from build123d import *

# Parameters (mm, degrees)
BOSS_EXTRUDE1_DEPTH      = 2
BOSS_EXTRUDE1_DEPTH_BACK = 2
SKETCH2_R                = 4
SKETCH2_R_2              = 2.5
SKETCH4_R                = 2
BOSS_EXTRUDE2_DEPTH      = 4
BOSS_EXTRUDE3_DEPTH      = 2


with BuildPart() as part:
    # Sketch2 → Boss-Extrude1 (new, two sides: drawn at the far end of the back side and taken through both)
    with BuildSketch(Plane(origin=(0, 0, 0), x_dir=(1, 0, 0), z_dir=(0, 1, 0)).offset(-BOSS_EXTRUDE1_DEPTH_BACK)):
        Polygon((-52.5, 10), (52.5, 10), (52.5, 0), (52.5, -2.5), (47.5, -7.5), (42.5, -7.5), (32.5, 2.5), (17.5, 2.5), (7.5, -7.5), (-7.5, -7.5), (-17.5, 2.5), (-32.5, 2.5), (-42.5, -7.5), (-47.5, -7.5), (-52.5, -2.5), (-52.5, 0), align=None)
        with Locations(Location((0, 0, 0), (0, 0, 270))):
            Circle(SKETCH2_R, mode=Mode.SUBTRACT)
        with Locations(Location((-45, 0, 0), (0, 0, 270))):
            Circle(SKETCH2_R_2, mode=Mode.SUBTRACT)
        with Locations(Location((45, 0, 0), (0, 0, 90))):
            Circle(SKETCH2_R_2, mode=Mode.SUBTRACT)
    extrude(amount=BOSS_EXTRUDE1_DEPTH + BOSS_EXTRUDE1_DEPTH_BACK)

    # Sketch4 → Boss-Extrude2 (add)
    with BuildSketch(Plane(origin=(0, 0, -10), x_dir=(-1, 0, 0), z_dir=(0, 0, -1))):
        Polygon((52.5, -8), (42.25, -8), (32.25, -18), (20.25, -18), (10.25, -8), (-10.25, -8), (-20.25, -18), (-32.25, -18), (-42.25, -8), (-52.5, -8), (-52.5, 8), (-42.25, 8), (-32.25, 18), (-20.25, 18), (-10.25, 8), (10.25, 8), (20.25, 18), (32.25, 18), (42.25, 8), (52.5, 8), align=None)
        with Locations((26.25, -10.674724776)):
            Circle(SKETCH4_R, mode=Mode.SUBTRACT)
        with Locations(Location((-26.25, -10.674724776, 0), (0, 0, 180))):
            Circle(SKETCH4_R, mode=Mode.SUBTRACT)
        with Locations((-26.25, 10.674724776)):
            Circle(SKETCH4_R, mode=Mode.SUBTRACT)
        with Locations(Location((26.25, 10.674724776, 0), (0, 0, 180))):
            Circle(SKETCH4_R, mode=Mode.SUBTRACT)
    extrude(amount=BOSS_EXTRUDE2_DEPTH)

    # Sketch5 → Boss-Extrude3 (add)
    with BuildSketch(Plane.ZY.offset(17.5)):
        Polygon((-10, 7), (-10, 2), (-2.5, 2), align=None)
        Polygon((-2.5, -2), (-10, -7), (-10, -2), align=None)
    boss_extrude3 = extrude(amount=-BOSS_EXTRUDE3_DEPTH)

    # Mirror1: Boss-Extrude3 across plane
    add(boss_extrude3.mirror(Plane(origin=(0, 0, 0), x_dir=(0, 0, 1), z_dir=(1, 0, 0))))


solid = part.part
Here's how the part is built. I have some questions about the finished solid (model axes, mm). A direction names the side the tool comes from. Give positions to 0.01 mm unless a question says otherwise; leave off trailing zeros. Write each loop counter-clockwise with the first axis right and the second up, starting at its lowest first coordinate (ties: lowest second). Pieces come first, ordered by that corner, then holes. Notation, with made-up numbers: (83.5, 7.25) -> (109.5, 7.25) arc R13 cw to (109.5, 28.25) -> close; hole circle Ø2 at (14, -15.75). An arc over 180 degrees is marked (long way). Use one line per item in the form item = value. Start each with the question number.
1. Imagine slicing it at A-A on x = -45. List the corners of the cut face in (y, z) for me, plus the area to 3 significant figures.
2. On a 3-axis mill with a long thin cutter (end or side, diameter ignored), from which of +Z, -Z, +X, -X, +Y, -Y can I reach the whole of each face in a straight line? I mean faces 5 (the face through (-39, 2, -3)), 6 (the face through (39, -2, -3)), 7 (the face through (25, 0, -2.5)). Say none if no direction works.
3. Imagine slicing it at D-D on x = -26.25. List the corners of the cut face in (y, z) for me, plus the area to 3 significant figures.
4. If I drill on L1, parallel to Y at x = -26.25, z = -11.3; L2, parallel to Z at x = 45, y = -1; L3, parallel to Z at x = -40, y = 4, over which ranges is the centre line in solid material (lowest first)?
5. Thinking about a two-plate mould opening in Y: for faces 1 (the face through (15.32, 13.07, -11.97)), 2 (the face through (45, 0, 7.5)), 3 (the face through (-16.514, -4.465, -6.198)), 4 (the face through (24.342, 11.275, -11.972)), which applies, +Y half, -Y half, draft (parallel to the pull), parting line (faces both ways), or undercut?
6. Imagine slicing it at C-C on z = 5.5. List the corners of the cut face in (x, y) for me, plus the area to 3 significant figures.
7. Imagine slicing it at B-B on y = -0.5. List the corners of the cut face in (x, z) for me.
8. Will these pins go through, and if not, where does the flat tip stop? pin 1 Ø1.5 at (y, z) = (-5.5, -7.5) entering from +X; pin 2 Ø13 at (x, y) = (-1.5, -10.5) entering from +Z; pin 3 Ø1.2 at (x, z) = (45.5, -12.5) entering from +Y; pin 4 Ø6 at (y, z) = (5.5, 2.5) entering from +X.
Entries:
q1.outline = (-8, -14) -> (8, -14) -> (8, -10) -> (2, -10) -> (2, -2.5) -> (-2, -2.5) -> (-2, -10) -> (-8, -10) -> close; (-2, 2.5) -> (2, 2.5) -> (2, 7.5) -> (-2, 7.5) -> close
q1.area = 114 mm²
q2.face_5 = +Z, -X, +Y
q2.face_6 = +Z, +X, -Y
q2.face_7 = +Z, +Y, -Y
q3.outline = (-18, -14) -> (-12.67, -14) -> (-12.67, -10) -> (-18, -10) -> close; (-8.67, -14) -> (8.67, -14) -> (8.67, -10) -> (2, -10) -> (2, -2.5) -> (-2, -2.5) -> (-2, -10) -> (-8.67, -10) -> close; (12.67, -14) -> (18, -14) -> (18, -10) -> (12.67, -10) -> close
q3.area = 142 mm²
q4.L1 = -18 to -12.67, -8.67 to 8.67, 12.67 to 18
q4.L2 = -14 to -2.5, 2.5 to 7.5
q4.L3 = -14 to -10
q5.face_1 = +Y half
q5.face_2 = draft
q5.face_3 = -Y half
q5.face_4 = undercut
q6.outline = (-49.5, -2) -> (-40.5, -2) -> (-40.5, 2) -> (-49.5, 2) -> close; (-9.5, -2) -> (9.5, -2) -> (9.5, 2) -> (-9.5, 2) -> close; (40.5, -2) -> (49.5, -2) -> (49.5, 2) -> (40.5, 2) -> close
q6.area = 148 mm²
q7.outline = (-52.5, -14) -> (52.5, -14) -> (52.5, 2.5) -> (47.5, 7.5) -> (42.5, 7.5) -> (32.5, -2.5) -> (17.5, -2.5) -> (7.5, 7.5) -> (-7.5, 7.5) -> (-17.5, -2.5) -> (-32.5, -2.5) -> (-42.5, 7.5) -> (-47.5, 7.5) -> (-52.5, 2.5) -> close; hole circle Ø5 at (-45, 0); hole circle Ø8 at (0, 0); hole circle Ø5 at (45, 0)
q8.pin_1 = 17.5
q8.pin_2 = -10
q8.pin_3 = 8
q8.pin_4 = through
